Verification items for the finished model (mm, model axes). A direction names the side the tool comes from. Round coordinates to 2 decimals unless told otherwise and drop trailing zeros. Write each loop counter-clockwise with the first axis right and the second up, starting at its lowest first coordinate (ties: lowest second). Pieces come first, ordered by that corner, then holes. Notation, with made-up numbers: M 63,58 L 76,58 A27 ccw 76,95 Z; hole C -23.5,-35.75 d2. An arc over 180 degrees is marked long. One line per item, written item: value. Start each with the question number.
Item 1: Section check D-D, the plane z = 0. State how many separate pieces and enclosed holes the cut face has, then the cut area to 3 significant figures.
Item 2: Thickness scan on probe 1 along X at (y, z) = (-34, 0); probe 2 along X at (y, z) = (0, 3); probe 3 along Y at (x, z) = (-7.5, 0). Record the ranges inside material, lowest first. Write a range as from..to.
Item 3: Section check A-A, the plane x = -32. Record the cut outline in (y, z), then the cut area to 3 significant figures.
Item 4: Draft check along Z on faces 4 (the face through (13.762, 15.505, 0.242)), 5 (the face through (0.642, -14.986, -0.14)), 6 (the face through (-1, -22, 10)), 7 (the face through (-1, -22, -10)). Enter one of: +Z half, -Z half, draft (parallel to the pull), parting line (faces both ways), or undercut.
Item 5: Section check B-B, the plane y = 21. Record the cut outline in (x, z).
Item 6: Gauge pin test, flat ends, axial feed: pin 1 (5 mm diameter, centred on y = 21, z = 0, fed in from +X); pin 2 (6.5 mm diameter, centred on y = 18.5, z = -4, fed in from -X); pin 3 (5.5 mm diameter, centred on y = 21, z = 0, fed in from -X). Record the tip position at first contact, or that the pin passes through.
Item 7: Section check C-C, the plane y = 11. Record the cut outline in (x, z), then the cut area to 3 significant figures.
Item 8: Tool access check on faces 1 (the face through (-22, -8, 0)), 2 (the face through (0, -41, 0)), 3 (the face through (4.9, 17.8, 0.1)). Record the directions out of +Z, -Z, +X, -X, +Y, -Y that give a thin tool (end or side, any length) a straight path to the whole face; none if there is none.
Autodesk Inventor part; units mm, degrees
ref_plane "to_bolt_XY" through (8.5, 21, 0) normal (1, 0, 0) x (0, 0, -1)
ref_plane "to_bolt_YZ" through (8.5, 21, 0) normal (0, 0, -1) x (0, 1, 0)
ref_plane "to_bolt_ZX" through (8.5, 21, 0) normal (0, 1, 0) x (1, 0, 0)
sketch "_____1" plane through (0, 0, 0) normal (0, 0, 1) x (1, 0, 0)
  line L0 (-40, -33) -> (-40, -42)
  line L1 (-40, -42) -> (-14, -42)
  arc A0 (-13, -41) -> (-14, -42) centre (-13, -42) ccw
  line L2 (-13, -41) -> (13, -41)
  arc A1 (14, -42) -> (13, -41) centre (13, -42) ccw
  line L3 (14, -42) -> (40, -42)
  line L4 (40, -42) -> (40, -33)
  arc A2 (40, -33) -> (39, -32) centre (39, -33) ccw
  line L5 (39, -32) -> (24, -32)
  arc A3 (22, -30) -> (24, -32) centre (24, -30) ccw
  line L6 (22, -30) -> (22, 13)
  arc A4 (22, 13) -> (7, 28) centre (7, 13) ccw
  line L7 (7, 28) -> (-7, 28)
  arc A5 (-7, 28) -> (-22, 13) centre (-7, 13) ccw
  line L8 (-22, 13) -> (-22, -30)
  arc A6 (-24, -32) -> (-22, -30) centre (-24, -30) ccw
  line L9 (-24, -32) -> (-39, -32)
  arc A7 (-39, -32) -> (-40, -33) centre (-39, -33) ccw
extrude "Extrusion1" add sketch "_____1" along normal mid plane 20
sketch "_____2" plane through (0, 0, 0) normal (0, 0, 1) x (1, 0, 0)
  arc A0 (-1.25, 14.9478) -> (1.25, 14.9478) centre (0, 0) ccw
  line L0 (1.25, 14.9478) -> (1.25, 70)
  line L1 (1.25, 70) -> (-1.25, 70)
  line L2 (-1.25, 70) -> (-1.25, 14.9478)
extrude "Extrusion2" cut sketch "_____2" along normal mid plane 20
sketch "_____3" plane through (0, 0, 0) normal (0, 1, 0) x (1, 0, 0)
  circle A0 centre (32, 0) radius 4.5
extrude "Extrusion3" cut sketch "_____3" against normal blind 42
sketch "_____4" plane through (0, 0, 0) normal (0, 1, 0) x (1, 0, 0)
  circle A0 centre (-32, 0) radius 4.5
extrude "Extrusion4" cut sketch "_____4" against normal blind 42
sketch "_____5" plane through (0, 0, 0) normal (0, 0, 1) x (1, 0, 0)
  line L0 (50, 21) -> (-50, 21)
  line L1 (0, 21) -> (0, 24.2)
  line L2 (0, 24.2) -> (8.5, 24.2)
  line L3 (8.5, 24.2) -> (8.5, 26.5)
  line L4 (8.5, 26.5) -> (22, 26.5)
  line L5 (22, 26.5) -> (22, 21)
  line L6 (22, 21) -> (0, 21)
revolve "Revolution1" cut sketch "_____5" angle 360 about axis through (50, 21, 0) along (1, 0, 0)
sketch "Sketch6" plane through (-1.25, 14.9478, 10) normal (1, 0, 0) x (0, 0, -1)
  point P0 (10, 6.0522)
hole "Hole1" at (-1.25, 21, 0) direction (-1, 0, 0) diameter 4.917 depth 20.75 countersink diameter 6 countersink angle 90
ref_plane "to_bolt_XY" through (8.5, 21, 0) normal (1, 0, 0) x (0, 0, -1)
ref_plane "to_bolt_YZ" through (8.5, 21, 0) normal (0, 0, -1) x (0, 1, 0)
ref_plane "to_bolt_ZX" through (8.5, 21, 0) normal (0, 1, 0) x (1, 0, 0)
properties part number "C-SHA30_b"
Response values:
1. separate pieces: 5
1. enclosed holes: 0
1. area: 2,140 mm2
2. probe 1: x = -40..-36.5, -27.5..27.5, 36.5..40
2. probe 2: x = -22..-15, 15..22
2. probe 3: y = -41..-12.99, 12.99..18.54, 23.46..27.99
3. outline: M -42,-10 L -32,-10 L -32,-4.5 L -42,-4.5 Z; M -42,4.5 L -32,4.5 L -32,10 L -42,10 Z
3. area: 110 mm2
4. face 4: undercut
4. face 5: draft
4. face 6: +Z half
4. face 7: -Z half
5. outline: M -19.69,-10 L -1.25,-10 L -1.25,-3 L -1.79,-2.46 L -19.69,-2.46 Z; M -19.69,2.46 L -1.79,2.46 L -1.25,3 L -1.25,10 L -19.69,10 Z; M 1.25,-10 L 19.69,-10 L 19.69,-5.5 L 8.5,-5.5 L 8.5,-3.2 L 1.25,-3.2 Z; M 1.25,3.2 L 8.5,3.2 L 8.5,5.5 L 19.69,5.5 L 19.69,10 L 1.25,10 Z
6. pin 1: stops at x = -1.75
6. pin 2: stops at x = -21.83
6. pin 3: stops at x = -21.05
7. outline: M -22,-10 L -10.2,-10 L -10.2,10 L -22,10 Z; M 10.2,-10 L 22,-10 L 22,10 L 10.2,10 Z
7. area: 472 mm2
8. face 1: +Z, -Z, -X, +Y
8. face 2: +Z, -Z, -Y
8. face 3: +X
